Part model, mm, in its own coordinate system. A direction names the side the tool comes from. Coordinates: 2 decimals unless noted, no trailing zeros. Loops run counter-clockwise (first coordinate to the right, second up) from the corner with the lowest first, then second, coordinate; pieces in that order, holes last. Notation, with made-up numbers: M -23,88 L 16,88 A21 cw 16,119 Z; hole C 28.5,-39.5 d4. An arc over 180 degrees is marked long. Answer as a JSON object with one key per item and string values. Group by question number.
1. Saw through at C-C on x = -11.5. Write the cut outline in (y, z).
2. Drill centre lines: L1, parallel to X at y = 2, z = 1.5; L2, parallel to Y at x = -13, z = -5.25; L3, parallel to Y at x = -25, z = 1. Where is each one in solid material? Low to high.
3. Drop flat-ended pins along their axis: pin 1 Ø1.5 at (y, z) = (7.5, -4.5) entering from +X; pin 2 Ø5 at (y, z) = (-5.5, 1) entering from +X; pin 3 Ø1.5 at (y, z) = (5.5, 0) entering from +X. Give the stop position or say it passes through.
4. Saw through at A-A on z = 2.5. Write the cut outline in (x, y), then the cut area to 3 significant figures.
5. 3-axis set-ups, long thin cutter, end or side, ignore diameter. For faces 4 (the face through (-0.5, -10.4, 7)), 5 (the face through (0, -10, 0)): which of +Z, -Z, +X, -X, +Y, -Y reach the whole face in a straight line?
6. Saw through at D-D on y = 28. Write the cut outline in (x, z), then the cut area to 3 significant figures.
7. Saw through at B-B on y = 10. Write the cut outline in (x, z), then the cut area to 3 significant figures.
8. Mould opens along X. For faces 1 (the face through (-8.78, 4.79, 0.1)), 2 (the face through (-1, -21.651, 0)), 3 (the face through (19.012, 10.371, 0.098)) say: released by +X, released by -X, zero draft, split by the parting line, or undercut.
from build123d import *

# Parameters (mm, degrees)
F1_DEPTH = 7


with BuildPart() as f1:
    # F0 (on Top) → F1 (new body, symmetric)
    with BuildSketch(Plane.XY):
        Polygon((0, 43.30127), (-37.5, -21.650635), (37.5, -21.650635), align=None)
        Polygon((0, 20), (17.320508, -10), (-17.320508, -10), align=None, mode=Mode.SUBTRACT)
    extrude(amount=F1_DEPTH, both=True)


solid = f1.part
Outcome:
{
 "1": {"outline": "M -21.65,-7 L -10,-7 L -10,7 L -21.65,7 Z; M 0.08,-7 L 23.38,-7 L 23.38,7 L 0.08,7 Z"},
 "2": {"L1": "x = -23.85 to -10.39, 10.39 to 23.85", "L2": "y = -21.65 to -10, -2.52 to 20.78", "L3": "y = -21.65 to 0"},
 "3": {"pin 1": "stops at x = 21.1", "pin 2": "stops at x = 29.62", "pin 3": "stops at x = 22.26"},
 "4": {"outline": "M -37.5,-21.65 L 37.5,-21.65 L 0,43.3 Z; hole M -17.32,-10 L 17.32,-10 L 0,20 Z", "area": "1,920 mm²"},
 "5": {"face 4": "+Z, +X, -X, +Y, -Y", "face 5": "+Z, -Z"},
 "6": {"outline": "M -8.83,-7 L 8.83,-7 L 8.83,7 L -8.83,7 Z", "area": "247 mm²"},
 "7": {"outline": "M -19.23,-7 L -5.77,-7 L -5.77,7 L -19.23,7 Z; M 5.77,-7 L 19.23,-7 L 19.23,7 L 5.77,7 Z", "area": "377 mm²"},
 "8": {"face 1": "undercut", "face 2": "zero draft", "face 3": "released by +X"}
}
